Could you check a few things on this model? Use its own coordinates, in mm. Face numbers are marked on the shaded views. A direction names the side the tool comes from. Round coordinates to 2 decimals unless told otherwise and drop trailing zeros. Write each loop counter-clockwise with the first axis right and the second up, starting at its lowest first coordinate (ties: lowest second). Pieces come first, ordered by that corner, then holes. Notation, with made-up numbers: (71.5, 45) - (101.5, 45) arc R27 ccw to (101.5, 67) - close; hole circle Ø1 at (28.5, 81). An arc over 180 degrees is marked (long way). Put each result on its own line as item: value.
from build123d import *

# Parameters (mm, degrees)
SKETCH1_R                   = 11.1125
BOSS_EXTRUDE1_DEPTH         = 3.175
SKETCH2_R                   = 3.175
BOSS_EXTRUDE2_DEPTH         = 25.4
F_44_0_086_DIAMETER_HOLE1_D = 2.1844


with BuildPart() as part:
    # Sketch1 → Boss-Extrude1 (new body)
    with BuildSketch(Plane.XY):
        Circle(SKETCH1_R)
    extrude(amount=BOSS_EXTRUDE1_DEPTH)

    # Sketch2 → Boss-Extrude2 (add)
    with BuildSketch(Plane.XY.offset(3.175)):
        Circle(SKETCH2_R)
    extrude(amount=BOSS_EXTRUDE2_DEPTH)

    # #44 (0.086) Diameter Hole1 (through all)
    with Locations(Plane.XY.offset(3.175)):
        with Locations((0, 8), (0, -8), (-8, 0), (8, 0)):
            Hole(F_44_0_086_DIAMETER_HOLE1_D / 2)


solid = part.part
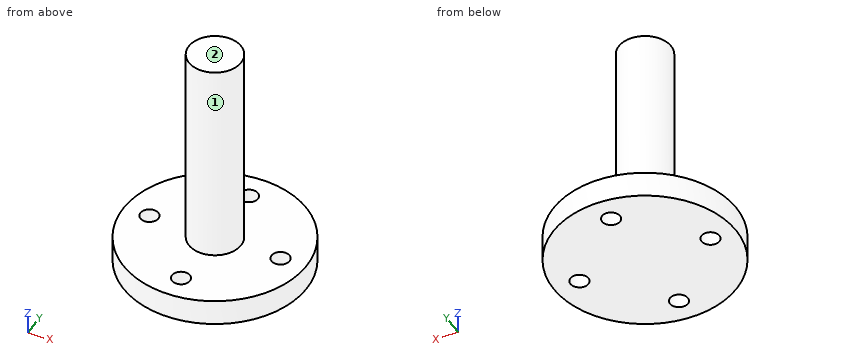
(1) Please list where these lines run through material, in increasing order: probe 1 along Y at (x, z) = (0, 1.4); probe 2 along Z at (x, y) = (1.5, -8) (3 decimals); probe 3 along Y at (x, z) = (8, 2.1). Write a range as from..to.
Values found:
probe 1: y = -11.11..-9.09, -6.91..6.91, 9.09..11.11
probe 2: z = 0..3.175
probe 3: y = -7.71..-1.09, 1.09..7.71
(2) I'm going to push flat-ended pins straight in: pin 1 (1.3 mm diameter, centred on x = 8, y = 0, fed in from +Z); pin 2 (6 mm diameter, centred on x = -2, z = 18, fed in from -Y) (3 decimals); pin 3 (1.5 mm diameter, centred on x = -5, y = 0, fed in from +Z) (3 decimals); pin 4 (10 mm diameter, centred on y = -1.5, z = 22, fed in from -X) (3 decimals). Where does each tip first touch, or does it pass through?
Values found:
pin 1: passes through
pin 2: stops at y = -3.175
pin 3: stops at z = 3.175
pin 4: stops at x = -3.175
(3) Imagine slicing it at C-C, the plane y = -8. List the corners of the cut face in (x, z) for me (3 decimals), then the cut area to 3 significant figures.
Values found:
outline: (-7.713, 0) - (-1.092, 0) - (-1.092, 3.175) - (-7.713, 3.175) - close; (1.092, 0) - (7.713, 0) - (7.713, 3.175) - (1.092, 3.175) - close
area: 42.0 mm^2
(4) Imagine slicing it at A-A, the plane y = 0. List the corners of the cut face in (x, z) for me (1 decimal).
Values found:
outline: (-11.1, 0) - (-9.1, 0) - (-9.1, 3.2) - (-11.1, 3.2) - close; (-6.9, 0) - (6.9, 0) - (6.9, 3.2) - (3.2, 3.2) - (3.2, 28.6) - (-3.2, 28.6) - (-3.2, 3.2) - (-6.9, 3.2) - close; (9.1, 0) - (11.1, 0) - (11.1, 3.2) - (9.1, 3.2) - close
(5) For the marked faces 1 and 2, which set-ups out of +Z, -Z, +X, -X, +Y, -Y let a thin tool reach every point of the face, with its end or its side?
Values found:
face 1: +Z
face 2: +Z, +X, -X, +Y, -Y
